```python
from build123d import *

# Parameters (mm, degrees)
SKETCH1_R             = 8.5
SKETCH1_R_2           = 7.5
BOSS_EXTRUDE1_DEPTH   = 6
SKETCH1_R_3           = 4.5
SKETCH1_R_4           = 3
BOSS_EXTRUDE1_2_DEPTH = 6
BOSS_EXTRUDE12_START  = 6
SKETCH1_4_R           = 9.5
SKETCH1_4_R_2         = 8.5
SKETCH1_4_R_3         = 7.5
SKETCH1_4_R_4         = 1.25
SKETCH1_4_R_5         = 4.5
BOSS_EXTRUDE12_DEPTH  = 2
SKETCH1_5_R           = 1.25
CUT_EXTRUDE2_DEPTH    = 7
CIRPATTERN1_COUNT     = 6


with BuildPart() as part:
    # Sketch1 → Boss-Extrude1 (new body, symmetric)
    with BuildSketch(Plane.XY):
        Circle(SKETCH1_R)
        Circle(SKETCH1_R_2, mode=Mode.SUBTRACT)
    extrude(amount=BOSS_EXTRUDE1_DEPTH, both=True)



with BuildPart() as body_2:
    # Sketch1 → Boss-Extrude1 2 (new body, symmetric)
    with BuildSketch(Plane.XY):
        Circle(SKETCH1_R_3)
        Circle(SKETCH1_R_4, mode=Mode.SUBTRACT)
    extrude(amount=BOSS_EXTRUDE1_2_DEPTH, both=True)


with BuildPart() as part_1:
    add(part.part)

    add(body_2.part)  # Boss-Extrude12 merges body 2
    # Sketch1<4> → Boss-Extrude12 (add)
    with BuildSketch(Plane.XY.offset(BOSS_EXTRUDE12_START)):
        Circle(SKETCH1_4_R)
        Circle(SKETCH1_4_R_2, mode=Mode.SUBTRACT)
        Circle(SKETCH1_4_R_3)
        with Locations((0, -6)):
            Circle(SKETCH1_4_R_4, mode=Mode.SUBTRACT)
        Circle(SKETCH1_4_R_5, mode=Mode.SUBTRACT)
    extrude(amount=-BOSS_EXTRUDE12_DEPTH)

    # Sketch1<5> → Cut-Extrude2 (cut, symmetric)
    with BuildSketch(Plane.XY):
        with Locations((0, -6)):
            Circle(SKETCH1_5_R)
    cut_extrude2 = extrude(amount=CUT_EXTRUDE2_DEPTH, both=True, mode=Mode.SUBTRACT)

    # CirPattern1: Cut-Extrude2 ×6 about axis
    cirpattern1_axis = Axis((0, 0, 0), (0, 0, 1))
    for i in range(1, CIRPATTERN1_COUNT):
        add(cut_extrude2.rotate(cirpattern1_axis, i * 360 / CIRPATTERN1_COUNT), mode=Mode.SUBTRACT)


solid = part_1.part
```
Geometry: final body of the model. Coordinates: model frame, mm. A direction names the side the tool comes from. Coordinates: 2 decimals unless noted, no trailing zeros. Write each loop counter-clockwise with the first axis right and the second up, starting at its lowest first coordinate (ties: lowest second). Pieces come first, ordered by that corner, then holes. Notation, with made-up numbers: M 14.25,-27 L 20.25,-27 A18 ccw 20.25,-18 Z; hole C 32.25,-32 d5. An arc over 180 degrees is marked long. Use CSV: the item, a comma, the result in double quotes. Start each with the question number.
1. First-contact query: P1, Ø5, axis at y = -1.5, z = -3, coming from the +X side; P2, Ø1, axis at y = 7.5, z = -3.5, coming from the +X side; P3, Ø1, axis at y = 1.5, z = 4.5, coming from the +X side. Flat tips, straight axial feed; report the tip coordinate or a pass-through.
2. Ray query, probe 1 along Y at (x, z) = (0, -0.5); probe 2 along Y at (x, z) = (-2, 0); probe 3 along X at (y, z) = (3.5, -2.75). Return the intervals inside material, ascending.
3. Cut plane A-A on y = 0. Return the cut outline in (x, z).
4. Cut plane C-C on z = -4.25. Return the cut outline in (x, y), plus the area to 3 significant figures.
5. Mould query, pull axis Y, two halves, no side actions, for faces 1 (the face through (-2.24, 2.24, 6)), 2 (the face through (-6.35, -2.52, 5.01)), 3 (the face through (4.38, -8.43, 5.01)). Classes: pulls with the +Y half, pulls with the -Y half, needs draft (parallel to the pull), parting line crosses it, or undercut.
6. Reachability of faces 4 (the face through (-7.493, 0.33, -1.07)), 5 (the face through (6.388, 3.375, 5.014)) from +Z, -Z, +X, -X, +Y, -Y: full face, straight path, thin tool, end or side. Return the list, or none.
7. Cut plane B-B on x = -2.25. Return the cut outline in (y, z), plus the area to 3 significant figures.
8. Cut plane D-D on y = 3.5. Return the cut outline in (x, z).
Entries:
1,P1,"x = 8.5"
1,P2,"x = 4.82"
1,P3,"x = 9.45"
2,probe 1,"-8.5 to -7.5, -4.5 to -3, 3 to 4.5, 7.5 to 8.5"
2,probe 2,"-8.26 to -7.23, -4.03 to -2.24, 2.24 to 4.03, 7.23 to 8.26"
2,probe 3,"-7.75 to -6.63, -2.83 to 2.83, 6.63 to 7.75"
3,outline,"M -9.5,4 L -8.5,4 L -8.5,-6 L -7.5,-6 L -7.5,4 L -4.5,4 L -4.5,-6 L -3,-6 L -3,6 L -9.5,6 Z; M 3,-6 L 4.5,-6 L 4.5,4 L 7.5,4 L 7.5,-6 L 8.5,-6 L 8.5,4 L 9.5,4 L 9.5,6 L 3,6 Z"
4,outline,"C 0,0 d17; C 0,0 d9; hole C 0,0 d15; hole C 0,0 d6"
4,area,"85.6 mm²"
5,face 1,"needs draft"
5,face 2,"undercut"
5,face 3,"parting line crosses it"
6,face 4,"-Z"
6,face 5,"+Z, -Z"
7,outline,"M -9.23,4 L -8.2,4 L -8.2,-6 L -7.15,-6 L -7.15,4 L -3.9,4 L -3.9,-6 L -1.98,-6 L -1.98,6 L -9.23,6 Z; M 1.98,-6 L 3.9,-6 L 3.9,4 L 7.15,4 L 7.15,-6 L 8.2,-6 L 8.2,4 L 9.23,4 L 9.23,6 L 1.98,6 Z"
7,area,"88.1 mm²"
8,outline,"M -8.83,4 L -7.75,4 L -7.75,-6 L -6.63,-6 L -6.63,4 L -6.34,4 L -6.34,6 L -8.83,6 Z; M -4.05,4 L -2.83,4 L -2.83,-6 L 2.83,-6 L 2.83,4 L 4.05,4 L 4.05,6 L -4.05,6 Z; M 6.34,4 L 6.63,4 L 6.63,-6 L 7.75,-6 L 7.75,4 L 8.83,4 L 8.83,6 L 6.34,6 Z"
